Autodesk Inventor part; units mm, degrees
ref_plane "YZ Plane" through (0, 0, 0) normal (1, 0, 0) x (0, 1, 0)
ref_plane "XZ Plane" through (0, 0, 0) normal (0, 1, 0) x (-1, 0, 0)
ref_plane "XY Plane" through (0, 0, 0) normal (0, 0, 1) x (1, 0, 0)
sketch "Szkic1" plane through (0, 0, 0) normal (0, 1, 0) x (-1, 0, 0)
  line L0 (7, -35.6103) -> (-8, -35.6103)
  line L1 (-8, -35.6103) -> (-8, -15.6103)
  line L2 (-8, -15.6103) -> (7, -15.6103)
  line L3 (7, -15.6103) -> (7, -35.6103)
  point P0 (0, 0)
  point P1 (2, -20.6103)
  dimension "d21" = 15
  dimension "d22" = 5
  dimension "d23" = 5
  dimension "d24" = 10
extrude "Wyciągnięcie proste3" add sketch "Szkic1" along normal blind 3
hole "Otwór2" at (-2, 0, -20.6103) direction (0, 1, 0) diameter 3 end through all
sketch "Szkic3" plane through (0, 3, 0) normal (0, 1, 0) x (1, 0, 0)
  line L0 (8, 35.6103) -> (8, 15.6103)
  line L1 (8, 35.6103) -> (5, 35.6103)
  line L2 (5, 35.6103) -> (5, 15.6103)
  line L3 (5, 15.6103) -> (8, 15.6103)
  line L4 (8, 15.6103) -> (8, 35.6103)
  point P0 (0, 0)
  dimension "d49" = 3
extrude "Wyciągnięcie proste4" add sketch "Szkic3" along normal blind 55.5
sketch "Szkic4" plane through (0, 58.5, 0) normal (0, 1, 0) x (1, 0, 0)
  line L0 (5, 15.6103) -> (5, 35.6103)
  line L1 (5, 35.6103) -> (-7, 35.6103)
  line L2 (-7, 35.6103) -> (-7, 15.6103)
  line L3 (-7, 15.6103) -> (5, 15.6103)
  circle A0 centre (-2, 20.6103) radius 1.5
  line L4 (8, 35.6103) -> (5, 35.6103)
  line L5 (5, 35.6103) -> (5, 15.6103)
  line L6 (5, 15.6103) -> (8, 15.6103)
  line L7 (8, 15.6103) -> (8, 35.6103)
  point P0 (0, 0)
extrude "Wyciągnięcie proste5" add sketch "Szkic4" along normal blind 3
sketch "Szkic5" plane through (8, 0, -15.6103) normal (1, 0, 0) x (0, 0, -1)
  line L0 (20, 0) -> (0, 0)
  line L1 (20, 0) -> (20, 61.5)
  line L2 (0, 61.5) -> (20, 61.5)
  line L3 (0, 0) -> (0, 61.5)
  point P0 (-15.6103, 0)
  point P1 (15, 40.75)
  point P2 (15, 20.75)
  dimension "d38" = 20
  dimension "d39" = 61.5
  dimension "d40" = 20.75
  dimension "d41" = 5
hole "Otwór3" at (8, 40.75, -30.6103) at (8, 20.75, -30.6103) direction (-1, 0, 0) diameter 3 end through all
Could you check a few things on this model? Use its own coordinates, in mm. A direction names the side the tool comes from. Coordinates: 2 decimals unless noted, no trailing zeros. Order: outer loops, then holes, each group sorted by start corner. A loop starts at its lowest first (then second) coordinate and runs counter-clockwise, first axis right, second up. Notation, with made-up numbers: M 84,28.5 L 119,28.5 A34 cw 119,67.5 Z; hole C 56.5,16 d6. An arc over 180 degrees is marked long. Use a Markdown table: item, result. Add a question column.
Q1. I want a section at C-C on x = -2. List the corners of the cut face in (y, z) for me, then the cut area to 3 significant figures.
Q2. I want a section at B-B on y = 40.75. List the corners of the cut face in (x, z) for me.
Q3. I want a section at A-A on x = 4. List the corners of the cut face in (y, z) for me, then the cut area to 3 significant figures.
Q4. I want a section at D-D on z = -23.75. List the corners of the cut face in (x, y) for me.
Q5. Which directions (+Z, -Z, +X, -X, +Y, -Y) give clear straight access to the entire face, cutting with the end or side of a thin tool? Please do faces 1 (the flat face through (-1, 3, -25)), 2 (the flat face through (-7, 1, -25)).
Q6. If I drill on L1, parallel to Y at x = -6, z = -29.75; L2, parallel to Z at x = 6.9, y = 20.75; L3, parallel to X at y = 17, z = -35, over which ranges is the centre line in solid material (lowest first)?
Q7. We'd pull the mould along X, two halves only. Please class faces 3 (the cylindrical face through (-2.325, 59.979, -22.075)), 4 (the cylindrical face through (6.48, 19.74, -29.5)), 5 (the flat face through (8, 30, -26)), 6 (the flat face through (5, 30, -26)): pulls with the +X half, pulls with the -X half, needs draft (parallel to the pull), parting line crosses it, or undercut.
Q8. I'm going to push flat-ended pins straight in: pin 1 (1.8 mm diameter, centred on y = 40.75, z = -30.61, fed in from +X); pin 2 (5 mm diameter, centred on y = 20.5, z = -19, fed in from -X). Where does each tip first touch, or does it pass through?
Checked values:
| question | item | result |
|---|---|---|
| 1 | outline | M 0,-35.61 L 3,-35.61 L 3,-22.11 L 0,-22.11 Z; M 0,-19.11 L 3,-19.11 L 3,-15.61 L 0,-15.61 Z; M 58.5,-35.61 L 61.5,-35.61 L 61.5,-22.11 L 58.5,-22.11 Z; M 58.5,-19.11 L 61.5,-19.11 L 61.5,-15.61 L 58.5,-15.61 Z |
| 1 | area | 102 mm² |
| 2 | outline | M 5,-35.61 L 8,-35.61 L 8,-32.11 L 5,-32.11 Z; M 5,-29.11 L 8,-29.11 L 8,-15.61 L 5,-15.61 Z |
| 3 | outline | M 0,-35.61 L 3,-35.61 L 3,-15.61 L 0,-15.61 Z; M 58.5,-35.61 L 61.5,-35.61 L 61.5,-15.61 L 58.5,-15.61 Z |
| 3 | area | 120 mm² |
| 4 | outline | M -7,0 L 8,0 L 8,61.5 L -7,61.5 L -7,58.5 L 5,58.5 L 5,3 L -7,3 Z |
| 5 | face 1 | +Z, -Z, -X |
| 5 | face 2 | +Z, -Z, -X, +Y, -Y |
| 6 | L1 | 0 to 3, 58.5 to 61.5 |
| 6 | L2 | -35.61 to -32.11, -29.11 to -15.61 |
| 6 | L3 | 5 to 8 |
| 7 | face 3 | undercut |
| 7 | face 4 | needs draft |
| 7 | face 5 | pulls with the +X half |
| 7 | face 6 | pulls with the -X half |
| 8 | pin 1 | through |
| 8 | pin 2 | x = 5 |
